from build123d import *

# Parameters (mm, degrees)
SKETCH1_R                  = 10.31875
BOSS_EXTRUDE1_DEPTH        = 3.175
SKETCH2_R                  = 6.35
BOSS_EXTRUDE2_DEPTH        = 6.35
SKETCH3_R                  = 3.175
CUT_EXTRUDE1_DEPTH         = 18.426383105
F_6_32_TAPPED_HOLE1_REACH  = 23.796
F_6_32_TAPPED_HOLE1_BORE_R = 1.35255


with BuildPart() as part:
    # Sketch1 → Boss-Extrude1 (new body)
    with BuildSketch(Plane.XY):
        Circle(SKETCH1_R)
    extrude(amount=BOSS_EXTRUDE1_DEPTH)

    # Sketch2 → Boss-Extrude2 (add)
    with BuildSketch(Plane.XY.offset(3.175)):
        Circle(SKETCH2_R)
    extrude(amount=BOSS_EXTRUDE2_DEPTH)

    # Sketch3 → Cut-Extrude1 (cut, through all)
    with BuildSketch(Plane(origin=(0, 0, 0), x_dir=(-1, 0, 0), z_dir=(0, 0, -1))):
        Circle(SKETCH3_R)
    extrude(amount=-CUT_EXTRUDE1_DEPTH, mode=Mode.SUBTRACT)

    # #6-32 Tapped Hole1 bore → #6-32 Tapped Hole1 (cut, up to next)
    with BuildSketch(Plane.ZY.offset(6.35), mode=Mode.PRIVATE) as f_6_32_tapped_hole1_sk1:
        with Locations((6.35, 0)):
            Circle(F_6_32_TAPPED_HOLE1_BORE_R)
    f_6_32_tapped_hole1_tool1 = extrude(f_6_32_tapped_hole1_sk1.sketch, amount=-F_6_32_TAPPED_HOLE1_REACH, mode=Mode.PRIVATE) & part.part
    add(f_6_32_tapped_hole1_tool1.solids().sort_by_distance((-6.35, 0, 6.35))[0], mode=Mode.SUBTRACT)


solid = part.part
Read the model definition and answer for the solid it produces. Units are mm, in the model's axes. A direction names the side the tool comes from. Give positions to 0.01 mm unless a question says otherwise; leave off trailing zeros. Write each loop counter-clockwise with the first axis right and the second up, starting at its lowest first coordinate (ties: lowest second). Pieces come first, ordered by that corner, then holes. Notation, with made-up numbers: (-7.75, 56.5) - (22.25, 56.5) arc R18 cw to (22.25, 87.5) - close; hole circle Ø6 at (69, 47.5). An arc over 180 degrees is marked (long way). Use CSV: the item, a comma, the result in double quotes. Start each with the question number.
(1) Find section D-D (y = 6). Give the vertices of the cut face in (x, z) (3 decimals).
(2) Given P1, Ø1.5, axis at y = -7.5, z = 4.5, coming from the +X side; P2, Ø5, axis at x = 4.5, z = 4.5, coming from the -Y side; P3, Ø1.5, axis at x = 1.5, z = 3.5, coming from the +Y side; P4, Ø4.5, axis at y = 0, z = 6.35, coming from the +X side, each flat-ended and moving along its own axis, determine where each tip first touches the part or whether it passes through.
(3) Consider line 1 along Y through (x, z) = (0, 2) (3 decimals); line 2 along Z through (x, y) = (-5.5, 0) (3 decimals); line 3 along Z through (x, y) = (8.25, -0.5) (3 decimals). Determine where each line is inside the solid, lowest interval first.
(4) Find section A-A (y = 0). Give the vertices of the cut face in (x, z) (3 decimals).
(5) For faces 4 (the cylindrical face through (6.057, 1.907, 6.306)), 5 (the flat face through (-2.4, 2.4, 0)), determine the directions among +Z, -Z, +X, -X, +Y, -Y from which every point of the face is accessible in a straight line to the end or side of a thin tool.
(6) Determine the mould class of faces 1 (the cylindrical face through (-4.6, 0.1, 5)), 2 (the flat face through (-2, 3, 9.525)), 3 (the cylindrical face through (-2.237, -10.073, 1.565)) for opening direction Z: +Z half, -Z half, draft (parallel to the pull), parting line (faces both ways), or undercut.
(7) Find section B-B (x = -5.5). Give the vertices of the cut face in (y, z) (3 decimals), plus the area to 3 significant figures.
Findings below:
1,outline,"(-8.395, 0) - (8.395, 0) - (8.395, 3.175) - (2.079, 3.175) - (2.079, 9.525) - (-2.079, 9.525) - (-2.079, 3.175) - (-8.395, 3.175) - close"
2,P1,"through"
2,P2,"y = -10.04"
2,P3,"y = 10.29"
2,P4,"x = 6.35"
3,line 1,"-10.319 to -3.175, 3.175 to 10.319"
3,line 2,"0 to 4.997, 7.703 to 9.525"
3,line 3,"0 to 3.175"
4,outline,"(-10.319, 0) - (-3.175, 0) - (-3.175, 4.997) - (-6.35, 4.997) - (-6.35, 3.175) - (-10.319, 3.175) - close; (-6.35, 7.703) - (-3.175, 7.703) - (-3.175, 9.525) - (-6.35, 9.525) - close; (3.175, 0) - (10.319, 0) - (10.319, 3.175) - (6.35, 3.175) - (6.35, 9.525) - (3.175, 9.525) - close"
5,face 4,"+Z"
5,face 5,"-Z, +X, -X, +Y, -Y"
6,face 1,"undercut"
6,face 2,"+Z half"
6,face 3,"draft"
7,outline,"(-8.731, 0) - (8.731, 0) - (8.731, 3.175) - (3.174, 3.175) - (3.174, 9.525) - (-3.174, 9.525) - (-3.174, 3.175) - (-8.731, 3.175) - close; hole circle Ø2.705 at (0, 6.35)"
7,area,"90.0 mm2"
